Work out the finished part from the listing and answer in its coordinate system (mm). A direction names the side the tool comes from. Round coordinates to 2 decimals unless told otherwise and drop trailing zeros. Write each loop counter-clockwise with the first axis right and the second up, starting at its lowest first coordinate (ties: lowest second). Pieces come first, ordered by that corner, then holes. Notation, with made-up numbers: (9, -12) - (35, -12) arc R33 ccw to (35, 24) - close; hole circle Ø8 at (80.5, 13.25). An arc over 180 degrees is marked (long way). Answer as a JSON object with one key per item and string values.
```python
from build123d import *

# Parameters (mm, degrees)
SKETCH_1_W          = 121.9
SKETCH_1_H          = 74.7
EXTRUDE_1_DEPTH     = 1.6
SKETCH_2_R          = 1.5
CUT_EXTRUDE_1_DEPTH = 1.6
FILLET_1_R          = 3
SKETCH_3_W          = 106.4
SKETCH_3_H          = 68.1
EXTRUDE_2_DEPTH     = 6.5
SKETCH_4_W          = 96
SKETCH_4_H          = 54.9
CUT_EXTRUDE_2_DEPTH = 0.1
SKETCH_6_W          = 13.573643903
SKETCH_6_H          = 15
CUT_EXTRUDE_3_DEPTH = 9.1
SKETCH_7_R          = 5
EXTRUDE_3_DEPTH     = 5.7


with BuildPart() as part:
    # 草图1 → 凸台-拉伸1 (new body)
    with BuildSketch(Plane.XY):
        Rectangle(SKETCH_1_W, SKETCH_1_H)
    extrude(amount=EXTRUDE_1_DEPTH)

    # 草图2 → 切除-拉伸1 (cut)
    with BuildSketch(Plane.XY.offset(1.6)):
        with Locations((-57.4, 33)):
            Circle(SKETCH_2_R)
        with Locations((-57.4, -33)):
            Circle(SKETCH_2_R)
        with Locations((57.4, -33)):
            Circle(SKETCH_2_R)
        with Locations((57.4, 33)):
            Circle(SKETCH_2_R)
    extrude(amount=-CUT_EXTRUDE_1_DEPTH, mode=Mode.SUBTRACT)

    # 圆角1
    fillet_1_edges = [part.edges().sort_by_distance(p)[0] for p in [
        (60.95, -37.35, 0.8),
        (-60.95, -37.35, 0.8),
        (-60.95, 37.35, 0.8),
        (60.95, 37.35, 0.8),
    ]]
    fillet(fillet_1_edges, radius=FILLET_1_R)

    # 草图3 → 凸台-拉伸2 (add)
    with BuildSketch(Plane.XY.offset(1.6)):
        Rectangle(SKETCH_3_W, SKETCH_3_H)
    extrude(amount=EXTRUDE_2_DEPTH)

    # 草图4 → 切除-拉伸2 (cut)
    with BuildSketch(Plane.XY.offset(8.1)):
        with Locations((0, 2.8)):
            Rectangle(SKETCH_4_W, SKETCH_4_H)
    extrude(amount=-CUT_EXTRUDE_2_DEPTH, mode=Mode.SUBTRACT)

    # 草图6 → 切除-拉伸3 (cut, through all)
    with BuildSketch(Plane(origin=(0, 0, 0), x_dir=(-1, 0, 0), z_dir=(0, 0, -1))):
        with Locations((63.536821952, -10.8)):
            Rectangle(SKETCH_6_W, SKETCH_6_H)
    extrude(amount=-CUT_EXTRUDE_3_DEPTH, mode=Mode.SUBTRACT)

    # 草图7 → 凸台-拉伸3 (add)
    with BuildSketch(Plane(origin=(0, 0, 0), x_dir=(-1, 0, 0), z_dir=(0, 0, -1))):
        with Locations((40.95, 25.35)):
            Circle(SKETCH_7_R)
    extrude(amount=EXTRUDE_3_DEPTH)


solid = part.part
```
Item 1: Determine the mould class of faces 1 (the flat face through (0, 36, 1.6)), 2 (the cylindrical face through (57.075, 31.536, 0.811)), 3 (the cylindrical face through (-37.265, 28.729, -2.81)) for opening direction X: pulls with the +X half, pulls with the -X half, needs draft (parallel to the pull), parting line crosses it, or undercut.
Results found:
{"face 1": "needs draft", "face 2": "undercut", "face 3": "parting line crosses it"}
Item 2: Each of these flat-tipped pins is pushed along its axis until it touches: P1, Ø0.5, axis at x = -60, z = 1, coming from the -Y side; P2, Ø3, axis at x = 12, y = -7.5, coming from the +Z side; P3, Ø1.5, axis at y = 5.5, z = -1, coming from the +X side; P4, Ø3, axis at y = -12, z = 4, coming from the +X side. Where does it stop, or does it pass through?
Results found:
{"P1": "y = -36.75", "P2": "z = 8", "P3": "through", "P4": "x = 53.2"}
Item 3: A cutting plane is placed at D-D (z = 5.5). Write down the section's boundary in (x, y).
Results found:
{"outline": "(-53.2, -34.05) - (53.2, -34.05) - (53.2, 34.05) - (-53.2, 34.05) - close"}
Item 4: Consider line 1 along Y through (x, z) = (57.4, 0.9); line 2 along Y through (x, z) = (-57.4, 0.55); line 3 along X through (y, z) = (-14, 0.75). Determine where each line is inside the solid, lowest interval first.
Results found:
{"line 1": "-37.35 to -34.5, -31.5 to 31.5, 34.5 to 37.35", "line 2": "-37.35 to -34.5, -31.5 to -18.3, -3.3 to 31.5, 34.5 to 37.35", "line 3": "-56.75 to 60.95"}
Item 5: A cutting plane is placed at B-B (y = 11). Write down the section's boundary in (x, z).
Results found:
{"outline": "(-60.95, 0) - (60.95, 0) - (60.95, 1.6) - (53.2, 1.6) - (53.2, 8.1) - (48, 8.1) - (48, 8) - (-48, 8) - (-48, 8.1) - (-53.2, 8.1) - (-53.2, 1.6) - (-60.95, 1.6) - close"}
Item 6: For faces 4 (the flat face through (53.2, 0, 5)), 5 (the flat face through (-1, 34.05, 5)), 6 (the flat face through (-53.2, 0, 5)), 7 (the flat face through (-1, -34.05, 5)), determine the directions among +Z, -Z, +X, -X, +Y, -Y from which every point of the face is accessible in a straight line to the end or side of a thin tool.
Results found:
{"face 4": "+Z, +X, +Y, -Y", "face 5": "+Z, +X, -X, +Y", "face 6": "+Z, -X, +Y, -Y", "face 7": "+Z, +X, -X, -Y"}
Item 7: A cutting plane is placed at A-A (x = -40.95). Write down the section's boundary in (y, z), and give its area (3 significant figures).
Results found:
{"outline": "(-37.35, 0) - (20.35, 0) - (20.35, -5.7) - (30.35, -5.7) - (30.35, 0) - (37.35, 0) - (37.35, 1.6) - (34.05, 1.6) - (34.05, 8.1) - (30.25, 8.1) - (30.25, 8) - (-24.65, 8) - (-24.65, 8.1) - (-34.05, 8.1) - (-34.05, 1.6) - (-37.35, 1.6) - close", "area": "614 mm²"}
Item 8: A cutting plane is placed at C-C (y = -11). Write down the section's boundary in (x, z), and give its area (3 significant figures).
Results found:
{"outline": "(-56.75, 0) - (60.95, 0) - (60.95, 1.6) - (53.2, 1.6) - (53.2, 8.1) - (48, 8.1) - (48, 8) - (-48, 8) - (-48, 8.1) - (-53.2, 8.1) - (-53.2, 1.6) - (-56.75, 1.6) - close", "area": "870 mm²"}
